The drawing under review shows one solid part. Ordinate dimensions are in mm from its lowest x, y, z. Round coordinates to 2 decimals unless told otherwise and drop trailing zeros. Order: outer loops, then holes, each group sorted by start corner. A loop starts at its lowest first (then second) coordinate and runs counter-clockwise, first axis right, second up. Notation, with made-up numbers: M -8,31 L 28,31 A8 cw 28,39 Z; hole C 88.5,31 d8. An arc over 180 degrees is marked long. Answer as a JSON object with one key per item and string values. Group by question number.
1) Insertion check: pin 1 Ø20.5 at (x, y) = (12.7, 12.7) entering from -Z; pin 2 Ø1.5 at (x, z) = (43.5, 1) entering from +Y (1 decimal). Each pin has a flat end and moves straight along its axis. Give the tip position at first contact, or say it passes through.
2) The part is to be moulded in two halves that separate along Y. For the marked faces 1, 2 and 3, say which applies: +Y half, -Y half, draft (parallel to the pull), parting line (faces both ways), or undercut.
3) Consider section B-B, the plane y = 12.7. Write out the cut boundary in (x, z).
4) Consider section A-A, the plane x = 12.7. Write out the cut boundary in (y, z).
5) Consider section C-C, the plane z = 4.5. Write out the cut boundary in (x, y), then the cut area to 3 significant figures.
6) To check wall thickness, follow line 1 (Y direction, x = 12.7, z = 2.5); line 2 (Y direction, x = 11.5, z = 3) (1 decimal); line 3 (X direction, y = 15, z = 5.5) (1 decimal). State the ranges of each line that lie inside material, in increasing order.
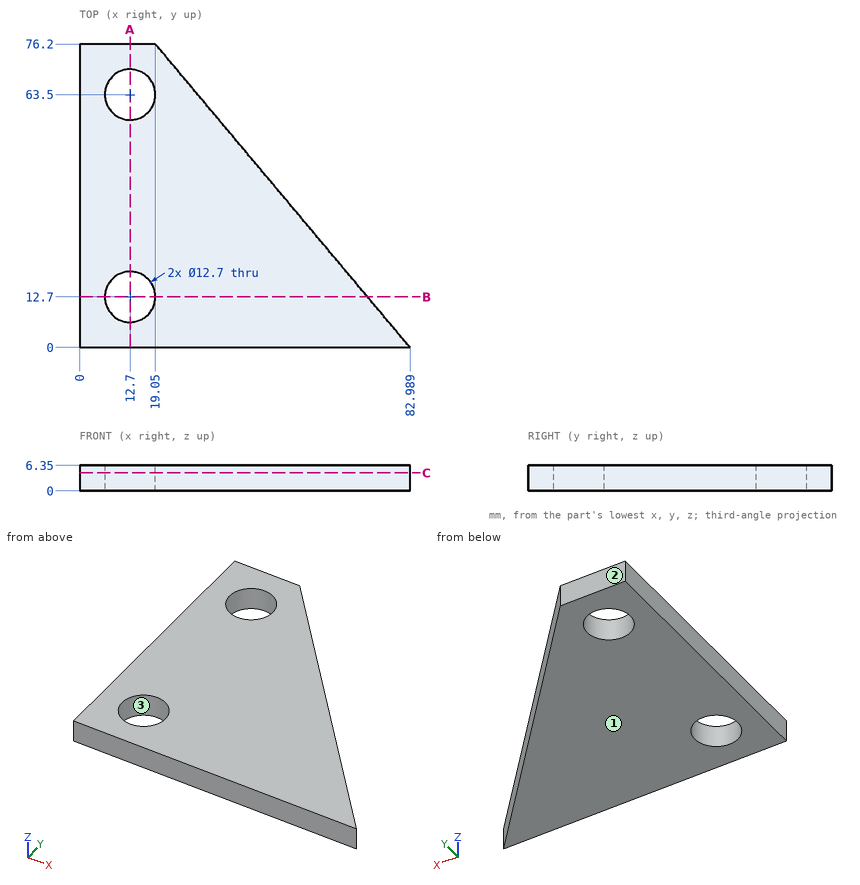
Results list:
{
 "1": {"pin 1": "z = 0", "pin 2": "y = 48"},
 "2": {"face 1": "draft", "face 2": "+Y half", "face 3": "undercut"},
 "3": {"outline": "M 0,0 L 6.35,0 L 6.35,6.35 L 0,6.35 Z; M 19.05,0 L 72.33,0 L 72.33,6.35 L 19.05,6.35 Z"},
 "4": {"outline": "M 0,0 L 6.35,0 L 6.35,6.35 L 0,6.35 Z; M 19.05,0 L 57.15,0 L 57.15,6.35 L 19.05,6.35 Z; M 69.85,0 L 76.2,0 L 76.2,6.35 L 69.85,6.35 Z"},
 "5": {"outline": "M 0,0 L 82.99,0 L 19.05,76.2 L 0,76.2 Z; hole C 12.7,12.7 d12.7; hole C 12.7,63.5 d12.7", "area": "3,630 mm^2"},
 "6": {"line 1": "0 to 6.35, 19.05 to 57.15, 69.85 to 76.2", "line 2": "0 to 6.5, 18.9 to 57.3, 69.7 to 76.2", "line 3": "0 to 6.8, 18.6 to 70.4"}
}
